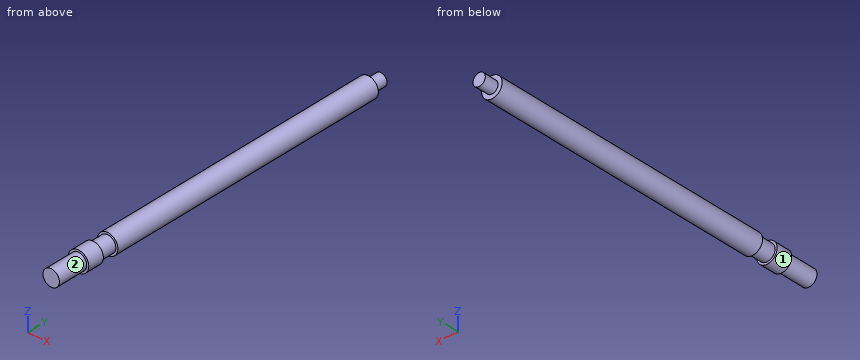
from build123d import *

# Parameters (mm, degrees)
SKETCH1_R           = 5
BOSS_EXTRUDE1_DEPTH = 143
SKETCH2_R           = 4
BOSS_EXTRUDE2_DEPTH = 8
BOSS_EXTRUDE3_START = 8
SKETCH3_R           = 5
BOSS_EXTRUDE3_DEPTH = 8
SKETCH4_R           = 4
BOSS_EXTRUDE4_DEPTH = 15
SKETCH5_R           = 3
BOSS_EXTRUDE5_DEPTH = 7


with BuildPart() as part:
    # Sketch1 → Boss-Extrude1 (new body)
    with BuildSketch(Plane(origin=(0, 0, 0), x_dir=(1, 0, 0), z_dir=(0, 1, 0))):
        with Locations(Location((0, 0, 0), (0, 0, 270))):
            Circle(SKETCH1_R)
    extrude(amount=BOSS_EXTRUDE1_DEPTH)

    # Sketch2 → Boss-Extrude2 (add)
    with BuildSketch(Plane.XZ):
        with Locations(Location((0, 0, 0), (0, 0, 270))):
            Circle(SKETCH2_R)
    extrude(amount=BOSS_EXTRUDE2_DEPTH)

    # Sketch3 → Boss-Extrude3 (add)
    with BuildSketch(Plane.XZ.offset(8).offset(BOSS_EXTRUDE3_START)):
        with Locations(Location((0, 0, 0), (0, 0, 90))):
            Circle(SKETCH3_R)
    extrude(amount=-BOSS_EXTRUDE3_DEPTH)

    # Sketch4 → Boss-Extrude4 (add)
    with BuildSketch(Plane.XZ.offset(16)):
        with Locations(Location((0, 0, 0), (0, 0, 270))):
            Circle(SKETCH4_R)
    extrude(amount=BOSS_EXTRUDE4_DEPTH)

    # Sketch5 → Boss-Extrude5 (add)
    with BuildSketch(Plane(origin=(0, 143, 0), x_dir=(1, 0, 0), z_dir=(0, 1, 0))):
        with Locations(Location((0, 0, 0), (0, 0, 270))):
            Circle(SKETCH5_R)
    extrude(amount=BOSS_EXTRUDE5_DEPTH)


solid = part.part
Could you check a few things on this model? Use its own coordinates, in mm. Face numbers are marked on the shaded views. A direction names the side the tool comes from. Give positions to 0.01 mm unless a question says otherwise; leave off trailing zeros. Write each loop counter-clockwise with the first axis right and the second up, starting at its lowest first coordinate (ties: lowest second). Pieces come first, ordered by that corner, then holes. Notation, with made-up numbers: (58, -14) -> (109, -14) arc R30 cw to (109, 9) -> close; hole circle Ø3 at (88, 58.5). An arc over 180 degrees is marked (long way). Answer as CSV lines item,"result". Start each with the question number.
(1) If we section it at C-C, the plane y = 4.5: Write out the boundary of the cut face in (x, z).
(2) Which directions (+Z, -Z, +X, -X, +Y, -Y) give clear straight access to the entire face, cutting with the end or side of a thin tool? Please do the marked faces 1 and 2.
(3) If we section it at A-A, the plane z = 0: Write out the boundary of the cut face in (x, y), and give its area (3 significant figures).
(4) Please list where these lines run through material, in increasing order: line 1 (Y direction, x = 3.25, z = 3.75); line 2 (Z direction, x = -4, y = 63); line 3 (Z direction, x = -0.5, y = 35.5).
(5) I'm going to push flat-ended pins straight in: pin 1 Ø1.5 at (x, y) = (-0.5, -7) entering from -Z; pin 2 Ø1 at (x, y) = (2.5, 82.5) entering from +Z. Where does each tip first touch, or does it pass through?
(6) If we section it at B-B, the plane x = 0: Write out the boundary of the cut face in (y, z), and give its area (3 significant figures).
Answer list:
1,outline,"circle Ø10 at (0, 0)"
2,face 1,"+Y, -Y"
2,face 2,"-Y"
3,outline,"(-5, -16) -> (-4, -16) -> (-4, -31) -> (4, -31) -> (4, -16) -> (5, -16) -> (5, -8) -> (4, -8) -> (4, 0) -> (5, 0) -> (5, 143) -> (3, 143) -> (3, 150) -> (-3, 150) -> (-3, 143) -> (-5, 143) -> (-5, 0) -> (-4, 0) -> (-4, -8) -> (-5, -8) -> close"
3,area,"1,740 mm^2"
4,line 1,"-16 to -8, 0 to 143"
4,line 2,"-3 to 3"
4,line 3,"-4.97 to 4.97"
5,pin 1,"z = -4"
5,pin 2,"z = 4.58"
6,outline,"(-31, -4) -> (-16, -4) -> (-16, -5) -> (-8, -5) -> (-8, -4) -> (0, -4) -> (0, -5) -> (143, -5) -> (143, -3) -> (150, -3) -> (150, 3) -> (143, 3) -> (143, 5) -> (0, 5) -> (0, 4) -> (-8, 4) -> (-8, 5) -> (-16, 5) -> (-16, 4) -> (-31, 4) -> close"
6,area,"1,740 mm^2"
